The drawing under review shows one solid part. Ordinate dimensions are in mm from its lowest x, y, z. Give positions to 0.01 mm unless a question says otherwise; leave off trailing zeros. Order: outer loops, then holes, each group sorted by start corner. A loop starts at its lowest first (then second) coordinate and runs counter-clockwise, first axis right, second up. Notation, with made-up numbers: (54, -25.75) -> (83, -25.75) arc R15 cw to (83, -20.75) -> close; hole circle Ø3 at (-20, 55.25). An arc over 180 degrees is marked (long way). Return JSON: item names as keys, results as strings. Group by question number.
1) Add section D-D (z = 17). Give the boundary of the cut face in (x, y).
2) Add section C-C (y = 1). Give the boundary of the cut face in (x, z).
3) Add section A-A (x = 40.5). Give the boundary of the cut face in (y, z).
4) The part is to be moulded in two halves that separate along Z. For the marked faces 1, 2 and 3, say which applies: released by +Z, released by -Z, zero draft, split by the parting line, or undercut.
5) To check wall thickness, follow line 1 along X through (y, z) = (7, 15.75). State the ranges of the line that lie inside material, in increasing order.
6) Add section B-B (z = 1). Give the boundary of the cut face in (x, y), then the cut area to 4 significant figures.
7) Insertion check: P1, Ø2, axis at y = 4, z = 7.5, coming from the +X side. The pin has a flat end and moves straight along its axis. Give the tip position at first contact, or say it passes through.
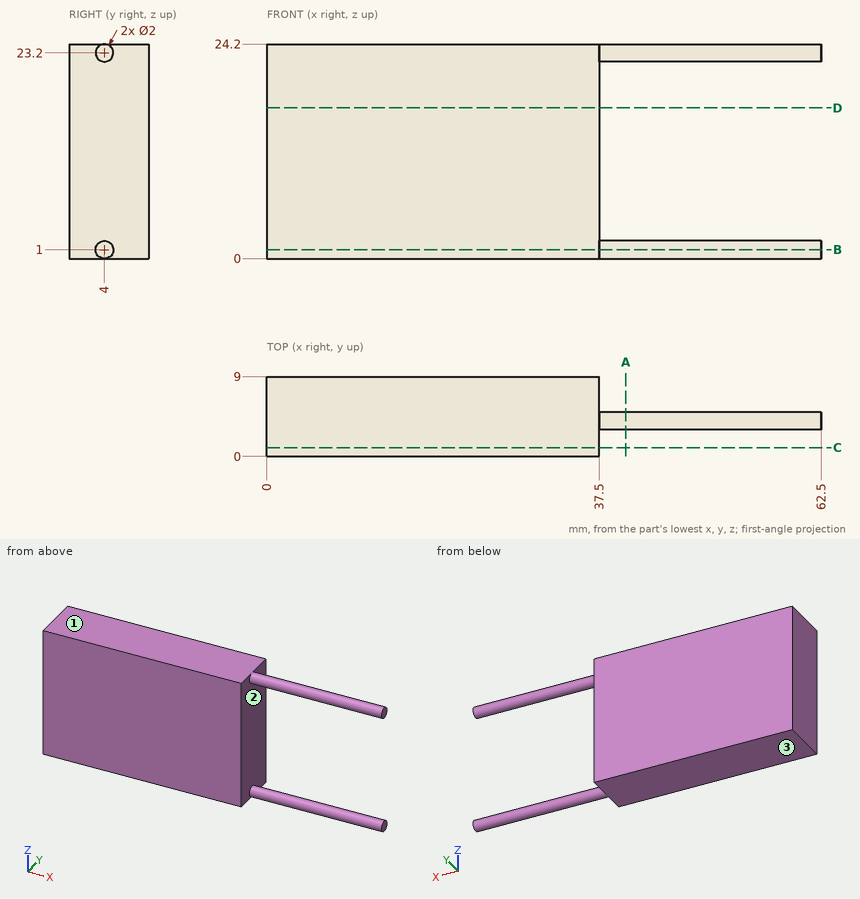
Evaluation:
{
 "1": {"outline": "(0, 0) -> (37.5, 0) -> (37.5, 9) -> (0, 9) -> close"},
 "2": {"outline": "(0, 0) -> (37.5, 0) -> (37.5, 24.2) -> (0, 24.2) -> close"},
 "3": {"outline": "circle Ø2 at (4, 1); circle Ø2 at (4, 23.2)"},
 "4": {"face 1": "released by +Z", "face 2": "undercut", "face 3": "released by -Z"},
 "5": {"line 1": "0 to 37.5"},
 "6": {"outline": "(0, 0) -> (37.5, 0) -> (37.5, 3) -> (62.5, 3) -> (62.5, 5) -> (37.5, 5) -> (37.5, 9) -> (0, 9) -> close", "area": "387.5 mm^2"},
 "7": {"P1": "x = 37.5"}
}
